from build123d import *

# Parameters (mm, degrees)
BOSS_EXTRUDE2_DEPTH          = 10
SKETCH5_R                    = 0.635
CUT_EXTRUDE1_DEPTH           = 10
CUT_EXTRUDE1_DRAFT           = 1.2
CUT_EXTRUDE1_PROFILE_2_DEPTH = 10
CUT_EXTRUDE1_PROFILE_2_DRAFT = 1.2


with BuildPart() as part:
    # Sketch2 → Boss-Extrude2 (new body)
    with BuildSketch(Plane(origin=(0, 0, 0), x_dir=(1, 0, 0), z_dir=(0, 1, 0))):
        with BuildLine():
            Line((0.055343897, 0.632583633), (0.075113859, 0.858555332))
            ThreePointArc((0.075113859, 0.858555332), (0.329887136, 1.190582332), (0.738477631, 1.1))
            Line((0.738477631, 1.1), (1.297487373, 0.540990258))
            ThreePointArc((1.297487373, 0.540990258), (1.619802906, 0.325625904), (2, 0.25))
            Line((2, 0.25), (6, 0.25))
            ThreePointArc((6, 0.25), (6.380197094, 0.325625904), (6.702512627, 0.540990258))
            Line((6.702512627, 0.540990258), (7.261522369, 1.1))
            ThreePointArc((7.261522369, 1.1), (7.670112864, 1.190582332), (7.924886141, 0.858555332))
            Line((7.924886141, 0.858555332), (7.944656103, 0.632583633))
            Line((7.944656103, 0.632583633), (7.944656103, -0.632583633))
            Line((7.944656103, -0.632583633), (7.924886141, -0.858555332))
            ThreePointArc((7.924886141, -0.858555332), (7.670112864, -1.190582332), (7.261522369, -1.1))
            Line((7.261522369, -1.1), (6.702512627, -0.540990258))
            ThreePointArc((6.702512627, -0.540990258), (6.380197094, -0.325625904), (6, -0.25))
            Line((6, -0.25), (2, -0.25))
            ThreePointArc((2, -0.25), (1.619802906, -0.325625904), (1.297487373, -0.540990258))
            Line((1.297487373, -0.540990258), (0.738477631, -1.1))
            ThreePointArc((0.738477631, -1.1), (0.329887136, -1.190582332), (0.075113859, -0.858555332))
            Line((0.075113859, -0.858555332), (0.055343897, -0.632583633))
            Line((0.055343897, -0.632583633), (0.055343897, 0.632583633))
        make_face()
    extrude(amount=BOSS_EXTRUDE2_DEPTH)


with BuildPart() as cut_extrude1_tool:
    # Sketch5 → Cut-Extrude1 (with draft: the straight prism first)
    with BuildSketch(Plane.XZ):
        Circle(SKETCH5_R)
    extrude(amount=-CUT_EXTRUDE1_DEPTH)
    # Cut-Extrude1: the draft: its side faces are tilted about the plane it starts from
    cut_extrude1_sides = [cut_extrude1_tool.faces().sort_by_distance(p)[0] for p in [
        (-0.635, 5, 0),
    ]]
    draft(cut_extrude1_sides, Plane.XZ, CUT_EXTRUDE1_DRAFT)


with BuildPart() as part_1:
    add(part.part)

    # Cut-Extrude1: cut by cut_extrude1_tool
    add(cut_extrude1_tool.part, mode=Mode.SUBTRACT)


with BuildPart() as cut_extrude1_profile_2_tool:
    # Sketch5 → Cut-Extrude1 profile 2 (with draft: the straight prism first)
    with BuildSketch(Plane.XZ):
        with Locations((8, 0)):
            Circle(SKETCH5_R)
    extrude(amount=-CUT_EXTRUDE1_PROFILE_2_DEPTH)
    # Cut-Extrude1 profile 2: the draft: its side faces are tilted about the plane it starts from
    cut_extrude1_profile_2_sides = [cut_extrude1_profile_2_tool.faces().sort_by_distance(p)[0] for p in [
        (7.365, 5, 0),
    ]]
    draft(cut_extrude1_profile_2_sides, Plane.XZ, CUT_EXTRUDE1_PROFILE_2_DRAFT)


with BuildPart() as part_2:
    add(part_1.part)

    # Cut-Extrude1 profile 2: cut by cut_extrude1_profile_2_tool
    add(cut_extrude1_profile_2_tool.part, mode=Mode.SUBTRACT)


solid = part_2.part
Build history of the part. All positions in model axes, mm. A direction names the side the tool comes from. Give positions to 0.01 mm unless a question says otherwise; leave off trailing zeros. Order: outer loops, then holes, each group sorted by start corner. A loop starts at its lowest first (then second) coordinate and runs counter-clockwise, first axis right, second up. Notation, with made-up numbers: M 8.25,-32 L 59.25,-32 A33 cw 59.25,4 Z; hole C -4.75,63 d2. An arc over 180 degrees is marked long. Use one line per item in the form item = value.
1) Drop flat-ended pins along their axis: pin 1 (1 mm diameter, centred on y = 7, z = -0.5, fed in from +X); pin 2 (4.5 mm diameter, centred on x = 5, y = 7, fed in from +Z); pin 3 (4.5 mm diameter, centred on x = 4.5, y = 3, fed in from -Z). Give the stop position or say it passes through.
Calculated:
pin_1 = 7.93
pin_2 = 1.09
pin_3 = -0.59
2) Saw through at C-C (y = 1.5). Give the cut face in (x, z).
Calculated:
outline = M 0.06,-0.66 L 0.08,-0.86 A0.39 ccw 0.74,-1.1 L 1.3,-0.54 A0.99 cw 2,-0.25 L 6,-0.25 A0.99 cw 6.7,-0.54 L 7.26,-1.1 A0.39 ccw 7.92,-0.86 L 7.94,-0.66 A0.67 cw 7.94,0.66 L 7.92,0.86 A0.39 ccw 7.26,1.1 L 6.7,0.54 A0.99 cw 6,0.25 L 2,0.25 A0.99 cw 1.3,0.54 L 0.74,1.1 A0.39 ccw 0.08,0.86 L 0.06,0.66 A0.67 cw Z
3) Saw through at A-A (y = 8.25). Give the cut face in (x, z).
Calculated:
outline = M 0.07,-0.8 L 0.08,-0.86 A0.39 ccw 0.74,-1.1 L 1.3,-0.54 A0.99 cw 2,-0.25 L 6,-0.25 A0.99 cw 6.7,-0.54 L 7.26,-1.1 A0.39 ccw 7.92,-0.86 L 7.93,-0.8 A0.81 cw 7.93,0.8 L 7.92,0.86 A0.39 ccw 7.26,1.1 L 6.7,0.54 A0.99 cw 6,0.25 L 2,0.25 A0.99 cw 1.3,0.54 L 0.74,1.1 A0.39 ccw 0.08,0.86 L 0.07,0.8 A0.81 cw Z
4) Tool access for faces 5 (the face through (0.738, 4.93, -0.015)), 6 (the face through (4, 10, 0)): list every direction of +Z, -Z, +X, -X, +Y, -Y with a clear straight run to the whole face (end or side of a thin tool).
Calculated:
face_5 = -X, +Y
face_6 = +Z, -Z, +X, -X, +Y
5) Saw through at B-B (x = 4). Give the cut face in (y, z), plus the area to 3 significant figures.
Calculated:
outline = M 0,-0.25 L 10,-0.25 L 10,0.25 L 0,0.25 Z
area = 5.00 mm2
6) Two-plate mould, pull along X, no slides. Class faces 1 (the face through (4, 5, 0.25)), 2 (the face through (4, 5, -0.25)), 3 (the face through (4, 0, 0)), 4 (the face through (7.262, 4.93, 0.015)): released by +X, released by -X, zero draft, split by the parting line, or undercut.
Calculated:
face_1 = undercut
face_2 = undercut
face_3 = zero draft
face_4 = released by +X
7) Probe probe 1 along Z at (x, y) = (3.5, 8); probe 2 along X at (y, z) = (1.5, -0.75); probe 3 along X at (y, z) = (5, 0.9). List the from-to ranges inside material, lowest first.
Calculated:
probe_1 = -0.25 to 0.25
probe_2 = 0.07 to 1.09, 6.91 to 7.93
probe_3 = 0.08 to 0.94, 7.06 to 7.92
